from build123d import *

# Parameters (mm, degrees)
SKETCH_1_W          = 190
SKETCH_1_H          = 130
SKETCH_1_R          = 2.5
EXTRUDE_1_DEPTH     = 5
FILLET_1_R          = 5
EXTRUDE_2_DEPTH     = 60
SKETCH_3_R          = 1
SKETCH_3_W          = 24
SKETCH_3_H          = 15
CUT_EXTRUDE_1_DEPTH = 10
CUT_EXTRUDE_2_DEPTH = 5


with BuildPart() as part:
    # 草圖1 → 填料-伸長1 (new body)
    with BuildSketch(Plane(origin=(0, 0, 0), x_dir=(1, 0, 0), z_dir=(0, 1, 0))):
        Rectangle(SKETCH_1_W, SKETCH_1_H)
        with Locations((-85, 55)):
            Circle(SKETCH_1_R, mode=Mode.SUBTRACT)
        with Locations((85, 55)):
            Circle(SKETCH_1_R, mode=Mode.SUBTRACT)
        with Locations((-85, -55)):
            Circle(SKETCH_1_R, mode=Mode.SUBTRACT)
        with Locations((85, -55)):
            Circle(SKETCH_1_R, mode=Mode.SUBTRACT)
    extrude(amount=EXTRUDE_1_DEPTH)

    # 圓角1
    fillet_1_edges = [part.edges().sort_by_distance(p)[0] for p in [
        (95, 2.5, 65),
        (-95, 2.5, 65),
        (-95, 2.5, -65),
        (95, 2.5, -65),
    ]]
    fillet(fillet_1_edges, radius=FILLET_1_R)

    # 草圖2 → 填料-伸長2 (add)
    with BuildSketch(Plane(origin=(0, 5, 0), x_dir=(1, 0, 0), z_dir=(0, 1, 0))):
        with BuildLine():
            Line((-80, 45), (-80, -45))
            ThreePointArc((-80, -45), (-78.535533906, -48.535533906), (-75, -50))
            Line((-75, -50), (75, -50))
            ThreePointArc((75, -50), (78.535533906, -48.535533906), (80, -45))
            Line((80, -45), (80, -5))
            Line((80, -5), (70, -5))
            Line((70, -5), (70, -35))
            ThreePointArc((70, -35), (68.535533906, -38.535533906), (65, -40))
            Line((65, -40), (-65, -40))
            ThreePointArc((-65, -40), (-68.535533906, -38.535533906), (-70, -35))
            Line((-70, -35), (-70, 35))
            ThreePointArc((-70, 35), (-68.535533906, 38.535533906), (-65, 40))
            Line((-65, 40), (65, 40))
            ThreePointArc((65, 40), (68.535533906, 38.535533906), (70, 35))
            Line((70, 35), (70, 5))
            Line((70, 5), (80, 5))
            Line((80, 5), (80, 45))
            ThreePointArc((80, 45), (78.535533906, 48.535533906), (75, 50))
            Line((75, 50), (-75, 50))
            ThreePointArc((-75, 50), (-78.535533906, 48.535533906), (-80, 45))
        make_face()
    extrude(amount=EXTRUDE_2_DEPTH)

    # 草圖3 → 除料-伸長1 (cut)
    with BuildSketch(Plane.ZY.offset(80)):
        with Locations((15, 47.5)):
            Circle(SKETCH_3_R)
        with Locations((-15, 47.5)):
            Circle(SKETCH_3_R)
        with Locations((0, 47.5)):
            Rectangle(SKETCH_3_W, SKETCH_3_H)
    extrude(amount=-CUT_EXTRUDE_1_DEPTH, mode=Mode.SUBTRACT)

    # 草圖4 → 除料-伸長2 (cut, symmetric)
    with BuildSketch(Plane(origin=(0, 30, 0), x_dir=(1, 0, 0), z_dir=(0, 1, 0))):
        with BuildLine():
            Line((-70, 45), (70, 45))
            ThreePointArc((70, 45), (73.535533906, 43.535533906), (75, 40))
            Line((75, 40), (75, -40))
            ThreePointArc((75, -40), (73.535533906, -43.535533906), (70, -45))
            Line((70, -45), (-70, -45))
            ThreePointArc((-70, -45), (-73.535533906, -43.535533906), (-75, -40))
            Line((-75, -40), (-75, 40))
            ThreePointArc((-75, 40), (-73.535533906, 43.535533906), (-70, 45))
        make_face()
        with BuildLine():
            Line((-65, 40), (65, 40))
            ThreePointArc((65, 40), (68.535533906, 38.535533906), (70, 35))
            Line((70, 35), (70, -35))
            ThreePointArc((70, -35), (68.535533906, -38.535533906), (65, -40))
            Line((65, -40), (-65, -40))
            ThreePointArc((-65, -40), (-68.535533906, -38.535533906), (-70, -35))
            Line((-70, -35), (-70, 35))
            ThreePointArc((-70, 35), (-68.535533906, 38.535533906), (-65, 40))
        make_face(mode=Mode.SUBTRACT)
    extrude(amount=CUT_EXTRUDE_2_DEPTH, both=True, mode=Mode.SUBTRACT)


solid = part.part
Work out the finished part from the listing and answer in its coordinate system (mm). A direction names the side the tool comes from. Round coordinates to 2 decimals unless told otherwise and drop trailing zeros. Write each loop counter-clockwise with the first axis right and the second up, starting at its lowest first coordinate (ties: lowest second). Pieces come first, ordered by that corner, then holes. Notation, with made-up numbers: (52, 33.25) -> (105, 33.25) arc R16 ccw to (105, 47.25) -> close; hole circle Ø11 at (80, -12). An arc over 180 degrees is marked (long way). Answer as CSV lines item,"result". Start each with the question number.
(1) The mould has two halves that part along X. Classify faces 6 (the flat face through (-70, 56, 0)), 7 (the flat face through (0, 65, -41)), 8 (the flat face through (-80, 35, -1)), 9 (the flat face through (80, 35, -25)): +X half, -X half, draft (parallel to the pull), parting line (faces both ways), or undercut.
(2) Find the intervals of material crossed by probe 1 along Z at (x, y) = (85, 1.3); probe 2 along Y at (x, z) = (-74, 15); probe 3 along Z at (x, y) = (-5.5, 12), in increasing order.
(3) A tool of negligible diameter and unlimited length cuts with its end or side. For faces 1 (the flat face through (-1, 2, -65)), 2 (the flat face through (-1, 50, -40)), 3 (the flat face through (-75, 47, -12)), 4 (the cylindrical face through (-73, 30, 44)), 5 (the cylindrical face through (93, 3, 64)), from which of +Z, -Z, +X, -X, +Y, -Y can it reach the whole face along a straight path? Write none if from no direction.
(4) Each of these flat-tipped pins is pushed along its axis until it touches: pin 1 (3 mm diameter, centred on y = 47.5, z = 15, fed in from -X); pin 2 (1.8 mm diameter, centred on y = 47.5, z = -15, fed in from -X); pin 3 (5 mm diameter, centred on x = 16, y = 35.5, fed in from -Z). Where does it stop, or does it pass through?
(5) The part is cut by section B-B, the plane x = 85. Give the vertices of the cut face in (y, z), then the cut area to 3 significant figures.
(6) The part is cut by section D-D, the plane z = 21. Give the vertices of the cut face in (x, y).
(7) The part is cut by section A-A, the plane z = 55. Give the vertices of the cut face in (x, y), then the cut area to 3 significant figures.
(8) The part is cut by section C-C, the plane x = -25.5. Give the vertices of the cut face in (y, z).
Output values:
1,face 6,"undercut"
1,face 7,"draft"
1,face 8,"-X half"
1,face 9,"+X half"
2,probe 1,"z = -65 to -57.5, -52.5 to 52.5, 57.5 to 65"
2,probe 2,"y = 0 to 25, 35 to 46.5, 48.5 to 65"
2,probe 3,"z = -50 to -40, 40 to 50"
3,face 1,"-Z, +X, -X, +Y, -Y"
3,face 2,"+Y"
3,face 3,"-X"
3,face 4,"none"
3,face 5,"+Z, +X, +Y, -Y"
4,pin 1,"stops at x = -80"
4,pin 2,"stops at x = 70"
4,pin 3,"stops at z = -50"
5,outline,"(0, -65) -> (5, -65) -> (5, -57.5) -> (0, -57.5) -> close; (0, -52.5) -> (5, -52.5) -> (5, 52.5) -> (0, 52.5) -> close; (0, 57.5) -> (5, 57.5) -> (5, 65) -> (0, 65) -> close"
5,area,"600 mm²"
6,outline,"(-95, 0) -> (95, 0) -> (95, 5) -> (80, 5) -> (80, 65) -> (70, 65) -> (70, 35) -> (75, 35) -> (75, 25) -> (70, 25) -> (70, 5) -> (-70, 5) -> (-70, 25) -> (-75, 25) -> (-75, 35) -> (-70, 35) -> (-70, 65) -> (-80, 65) -> (-80, 5) -> (-95, 5) -> close"
7,outline,"(-95, 0) -> (-87.5, 0) -> (-87.5, 5) -> (-95, 5) -> close; (-82.5, 0) -> (82.5, 0) -> (82.5, 5) -> (-82.5, 5) -> close; (87.5, 0) -> (95, 0) -> (95, 5) -> (87.5, 5) -> close"
7,area,"900 mm²"
8,outline,"(0, -65) -> (5, -65) -> (5, -50) -> (65, -50) -> (65, -40) -> (35, -40) -> (35, -45) -> (25, -45) -> (25, -40) -> (5, -40) -> (5, 40) -> (25, 40) -> (25, 45) -> (35, 45) -> (35, 40) -> (65, 40) -> (65, 50) -> (5, 50) -> (5, 65) -> (0, 65) -> close"
